The listing builds one solid part. Answer for the finished solid, in the listing's coordinates (mm). A direction names the side the tool comes from. Coordinates: 2 decimals unless noted, no trailing zeros. Write each loop counter-clockwise with the first axis right and the second up, starting at its lowest first coordinate (ties: lowest second). Pieces come first, ordered by that corner, then holes.
from build123d import *

# Parameters (mm, degrees)
F0_R     = 12.5
F0_R_2   = 2.3
F1_DEPTH = 1.56
F2_DEPTH = 6.2
F3_DEPTH = 7.48
F4_DEPTH = 2.5
F6_DEPTH = 5
F7_COUNT = 4


with BuildPart() as f1:
    # F0 (on Top) → F1 (new body)
    with BuildSketch(Plane.XY):
        with BuildLine():
            ThreePointArc((10.9357430539, -9.5215294916), (13.5797325872, -5.083390882), (14.5, 0))
            ThreePointArc((14.5, 0), (13.5797325872, 5.083390882), (10.9357430539, 9.5215294916))
            ThreePointArc((10.9357430539, 9.5215294916), (10.2530483272, 10.2530483272), (9.5215294916, 10.9357430539))
            ThreePointArc((9.5215294916, 10.9357430539), (0, 14.5), (-9.5215294916, 10.9357430539))
            ThreePointArc((-9.5215294916, 10.9357430539), (-10.2530483272, 10.2530483272), (-10.9357430539, 9.5215294916))
            ThreePointArc((-10.9357430539, 9.5215294916), (-14.5, 0), (-10.9357430539, -9.5215294916))
            ThreePointArc((-10.9357430539, -9.5215294916), (-10.2530483272, -10.2530483272), (-9.5215294916, -10.9357430539))
            ThreePointArc((-9.5215294916, -10.9357430539), (0, -14.5), (9.5215294916, -10.9357430539))
            ThreePointArc((9.5215294916, -10.9357430539), (10.2530483272, -10.2530483272), (10.9357430539, -9.5215294916))
        make_face()
        Circle(F0_R, mode=Mode.SUBTRACT)
        Circle(F0_R)
        with Locations((-9, 0)):
            Circle(F0_R_2, mode=Mode.SUBTRACT)
        with BuildLine():
            ThreePointArc((-5.12, 0), (0, 5.12), (5.12, 0))
            ThreePointArc((5.12, 0), (0, -5.12), (-5.12, 0))
        make_face(mode=Mode.SUBTRACT)
        with BuildLine():
            ThreePointArc((11.3, 0), (9, -2.3), (6.7, 0))
            ThreePointArc((6.7, 0), (9, 2.3), (11.3, 0))
        make_face(mode=Mode.SUBTRACT)
        with Locations((-9, 0)):
            Circle(F0_R_2)
        with BuildLine():
            ThreePointArc((11.3, 0), (9, 2.3), (6.7, 0))
            ThreePointArc((6.7, 0), (9, -2.3), (11.3, 0))
        make_face()
    extrude(amount=F1_DEPTH)

    # F0 (on Top) → F2 (join)
    with BuildSketch(Plane.XY):
        with BuildLine():
            ThreePointArc((10.9357430539, -9.5215294916), (13.5797325872, -5.083390882), (14.5, 0))
            ThreePointArc((14.5, 0), (13.5797325872, 5.083390882), (10.9357430539, 9.5215294916))
            ThreePointArc((10.9357430539, 9.5215294916), (10.2530483272, 10.2530483272), (9.5215294916, 10.9357430539))
            ThreePointArc((9.5215294916, 10.9357430539), (0, 14.5), (-9.5215294916, 10.9357430539))
            ThreePointArc((-9.5215294916, 10.9357430539), (-10.2530483272, 10.2530483272), (-10.9357430539, 9.5215294916))
            ThreePointArc((-10.9357430539, 9.5215294916), (-14.5, 0), (-10.9357430539, -9.5215294916))
            ThreePointArc((-10.9357430539, -9.5215294916), (-10.2530483272, -10.2530483272), (-9.5215294916, -10.9357430539))
            ThreePointArc((-9.5215294916, -10.9357430539), (0, -14.5), (9.5215294916, -10.9357430539))
            ThreePointArc((9.5215294916, -10.9357430539), (10.2530483272, -10.2530483272), (10.9357430539, -9.5215294916))
        make_face()
        Circle(F0_R, mode=Mode.SUBTRACT)
    extrude(amount=F2_DEPTH)

    # F0 (on Top) → F3 (join)
    with BuildSketch(Plane.XY):
        with BuildLine():
            Line((-13.2691954318, -14.6834089942), (-9.5215294916, -10.9357430539))
            ThreePointArc((-9.5215294916, -10.9357430539), (-10.2530483272, -10.2530483272), (-10.9357430539, -9.5215294916))
            Line((-10.9357430539, -9.5215294916), (-14.6834089942, -13.2691954318))
            Line((-14.6834089942, -13.2691954318), (-13.2691954318, -14.6834089942))
        make_face()
        with BuildLine():
            ThreePointArc((-10.9357430539, 9.5215294916), (-10.2530483272, 10.2530483272), (-9.5215294916, 10.9357430539))
            Line((-9.5215294916, 10.9357430539), (-13.2691954318, 14.6834089942))
            Line((-13.2691954318, 14.6834089942), (-14.6834089942, 13.2691954318))
            Line((-14.6834089942, 13.2691954318), (-10.9357430539, 9.5215294916))
        make_face()
        with BuildLine():
            ThreePointArc((9.5215294916, 10.9357430539), (10.2530483272, 10.2530483272), (10.9357430539, 9.5215294916))
            Line((10.9357430539, 9.5215294916), (14.6834089942, 13.2691954318))
            Line((14.6834089942, 13.2691954318), (13.2691954318, 14.6834089942))
            Line((13.2691954318, 14.6834089942), (9.5215294916, 10.9357430539))
        make_face()
        with BuildLine():
            Line((14.6834089942, -13.2691954318), (10.9357430539, -9.5215294916))
            ThreePointArc((10.9357430539, -9.5215294916), (10.2530483272, -10.2530483272), (9.5215294916, -10.9357430539))
            Line((9.5215294916, -10.9357430539), (13.2691954318, -14.6834089942))
            Line((13.2691954318, -14.6834089942), (14.6834089942, -13.2691954318))
        make_face()
    extrude(amount=F3_DEPTH)

    # F0 (on Top) → F4 (join)
    with BuildSketch(Plane.XY):
        with Locations((-9, 0)):
            Circle(F0_R_2)
        with BuildLine():
            ThreePointArc((11.3, 0), (9, 2.3), (6.7, 0))
            ThreePointArc((6.7, 0), (9, -2.3), (11.3, 0))
        make_face()
    extrude(amount=-F4_DEPTH)

    # F7: F6 ×4 about axis
    f7_axis = Axis((0, 0, 6.2), (0, 0, 1))


with BuildPart() as f6:
    # F5 (on face) → F6 (new body)
    with BuildSketch(Plane(origin=(0.7071067812, -0.7071067812, 0), x_dir=(0.7071067812, 0.7071067812, 0), z_dir=(0.7071067812, -0.7071067812, 0))):
        Polygon((-14.4654761415, 7.48), (-19.7654761415, 7.48), (-14.4654761415, 6.17), (-14.4654761415, 6.2), align=None)
    extrude(amount=-F6_DEPTH)


with BuildPart() as f1_1:
    add(f1.part)
    for i in range(1, F7_COUNT):
        add(f6.part.rotate(f7_axis, i * 360 / F7_COUNT), mode=Mode.SUBTRACT)

    # F7#seed: cut F6
    add(f6.part, mode=Mode.SUBTRACT)


solid = f1_1.part
1. Find the intervals of material crossed by L1, parallel to X at y = 0, z = 0.8; L2, parallel to X at y = 0, z = 5; L3, parallel to Y at x = -11.5, z = 1.75, in increasing order.
Results found:
L1: x = -14.5 to -5.12, 5.12 to 14.5
L2: x = -14.5 to -12.5, 12.5 to 14.5
L3: y = -12.91 to -10.09, -8.83 to -4.9, 4.9 to 8.83, 10.09 to 12.91
2. Section A-A on z = 1 is taken. Give the vertices of the cut face in (x, y).
Results found:
outline: (-14.68, -13.27) - (-13.27, -14.68) - (-9.52, -10.94) arc R14.5 ccw to (9.52, -10.94) - (13.27, -14.68) - (14.68, -13.27) - (10.94, -9.52) arc R14.5 ccw to (10.94, 9.52) - (14.68, 13.27) - (13.27, 14.68) - (9.52, 10.94) arc R14.5 ccw to (-9.52, 10.94) - (-13.27, 14.68) - (-14.68, 13.27) - (-10.94, 9.52) arc R14.5 ccw to (-10.94, -9.52) - close; hole circle Ø10.24 at (0, 0)
3. Section C-C on x = 0 is taken. Give the vertices of the cut face in (y, z).
Results found:
outline: (-14.5, 0) - (-5.12, 0) - (-5.12, 1.56) - (-12.5, 1.56) - (-12.5, 6.2) - (-14.5, 6.2) - close; (5.12, 0) - (14.5, 0) - (14.5, 6.2) - (12.5, 6.2) - (12.5, 1.56) - (5.12, 1.56) - close
4. Flat-ended cylindrical pins translate along their axes: P1, Ø4, axis at x = -4.5, y = 10.5, coming from the +Z side; P2, Ø4, axis at x = -2.5, z = 2, coming from the -Y side; P3, Ø1, axis at x = -11, y = 11.5, coming from the -Z side; P4, Ø9, axis at x = 4, y = 4, coming from the -Z side. Find the tip coordinate at first contact, or state that the pin passes through.
Results found:
P1: stops at z = 6.2
P2: stops at y = -14.49
P3: stops at z = 0
P4: stops at z = -2.5
5. A tool of negligible diameter and unlimited length cuts with its end or side. For faces 1 (the flat face through (-11, 7, 6.2)), 2 (the flat face through (-12.783, -11.369, 3.688)), 3 (the flat face through (-11.422, -12.836, 3.688)), from which of +Z, -Z, +X, -X, +Y, -Y can it reach the whole face along a straight path? Write none if from no direction.
Results found:
face 1: +Z
face 2: +Z, -Z, -X
face 3: +Z, -Z, -Y
6. Section B-B on y = 0 is taken. Give the vertices of the cut face in (x, z), then the cut area to 3 significant figures.
Results found:
outline: (-14.5, 0) - (-11.3, 0) - (-11.3, -2.5) - (-6.7, -2.5) - (-6.7, 0) - (-5.12, 0) - (-5.12, 1.56) - (-12.5, 1.56) - (-12.5, 6.2) - (-14.5, 6.2) - close; (5.12, 0) - (6.7, 0) - (6.7, -2.5) - (11.3, -2.5) - (11.3, 0) - (14.5, 0) - (14.5, 6.2) - (12.5, 6.2) - (12.5, 1.56) - (5.12, 1.56) - close
area: 70.8 mm2
